```python
from build123d import *

# Parameters (mm, degrees)
SKETCH_1_W      = 56.1
SKETCH_1_H      = 8
SKETCH_1_R      = 1.5
EXTRUDE_1_DEPTH = 8
EXTRUDE_5_DEPTH = 8
EXTRUDE_6_DEPTH = 8


with BuildPart() as part:
    # 草图1 → 凸台-拉伸1 (new body)
    with BuildSketch(Plane.XY):
        with Locations((28.05, -4)):
            Rectangle(SKETCH_1_W, SKETCH_1_H)
        with Locations((5, -4)):
            Circle(SKETCH_1_R, mode=Mode.SUBTRACT)
        with Locations(Location((51.1, -4, 0), (0, 0, 180))):
            Circle(SKETCH_1_R, mode=Mode.SUBTRACT)
    extrude(amount=EXTRUDE_1_DEPTH)

    # 草图3 → 凸台-拉伸5 (add)
    with BuildSketch(Plane(origin=(0, 0, 0), x_dir=(-1, 0, 0), z_dir=(0, 0, -1))):
        with BuildLine():
            Line((-9.271136129, 3.747804008), (-22.014574203, 0))
            Line((-22.014574203, 0), (0, 0))
            ThreePointArc((0, 0), (250.320675472, 168.809291774), (500.641350944, 0))
            Line((500.641350944, 0), (509.912487072, 0))
            Line((509.912487072, 0), (509.912487072, 3.747804008))
            ThreePointArc((509.912487072, 3.747804008), (250.320675472, 178.809291774), (-9.271136129, 3.747804008))
        make_face()
    extrude(amount=-EXTRUDE_5_DEPTH)

    # 草图4 → 凸台-拉伸6 (add)
    with BuildSketch(Plane(origin=(0, 0, 0), x_dir=(-1, 0, 0), z_dir=(0, 0, -1))):
        with BuildLine():
            ThreePointArc((152.808242493, 161.280862452), (28.754408722, 106.028077563), (-56.1, 0))
            Line((-56.1, 0), (-39.057287102, 0))
            ThreePointArc((-39.057287102, 0), (9.399846723, 74.751796663), (83.727278113, 123.857375428))
            ThreePointArc((83.727278113, 123.857375428), (116.948632862, 145.004129758), (152.808242493, 161.280862452))
        make_face()
    extrude(amount=-EXTRUDE_6_DEPTH)


solid = part.part
```
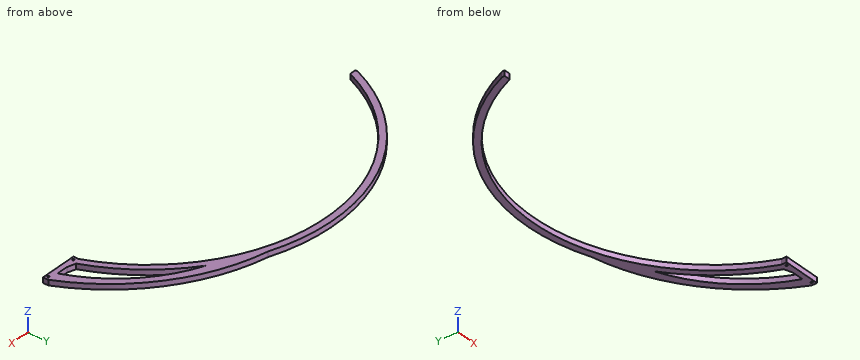
Read the model definition and answer for the solid it produces. Units are mm, in the model's axes. Give positions to 0.01 mm unless a question says otherwise; leave off trailing zeros. Order: outer loops, then holes, each group sorted by start corner. A loop starts at its lowest first (then second) coordinate and runs counter-clockwise, first axis right, second up.
(1) Find section D-D (y = 105). Give the vertices of the cut face in (x, z), plus the area to 3 significant figures.
(2) Find section B-B (y = 57). Give the vertices of the cut face in (x, z), plus the area to 3 significant figures.
(3) Find section A-A (z = 2.5). Give the vertices of the cut face in (x, y), plus the area to 3 significant figures.
(4) Given pin 1 (2.5 mm diameter, centred on y = -5.5, z = 4, fed in from -X); pin 2 (1 mm diameter, centred on y = 132.5, z = 4.5, fed in from +X); pin 3 (1.5 mm diameter, centred on y = 128.5, z = 6.5, fed in from -X); pin 4 (1.8 mm diameter, centred on x = 51.1, y = -4, fed in from +Z), each flat-ended and moving along its own axis, determine where each tip first touches the part or whether it passes through.
(5) Find section C-C (x = -88.5). Give the vertices of the cut face in (y, z), plus the area to 3 significant figures.
(6) Straight lines are drawn through the part: L1, parallel to X at y = 95.5, z = 3.75; L2, parallel to Y at x = 5, z = 4.75; L3, parallel to X at y = 50.5, z = 2. For each, find the intervals that lie inside material, in ascending order.
Result sheet:
1. outline: (-439.76, 0) - (-424.63, 0) - (-424.63, 8) - (-439.76, 8) - close; (-76.01, 0) - (-60.89, 0) - (-60.89, 8) - (-76.01, 8) - close; (-46.88, 0) - (-27.43, 0) - (-27.43, 8) - (-46.88, 8) - close
1. area: 398 mm2
2. outline: (-481.35, 0) - (-469.13, 0) - (-469.13, 8) - (-481.35, 8) - close; (-31.52, 0) - (-19.29, 0) - (-19.29, 8) - (-31.52, 8) - close; (6.38, 0) - (20.9, 0) - (20.9, 8) - (6.38, 8) - close
2. area: 312 mm2
3. outline: (-509.91, 0) - (-500.64, 0) arc R270 cw to (0, 0) - (0, -8) - (56.1, -8) - (56.1, 0) arc R287.5 ccw to (-152.81, 161.28) arc R280 ccw to (-509.91, 3.75) - close; hole (-83.73, 123.86) arc R280 cw to (9.27, 3.75) - (22.01, 0) - (39.06, 0) arc R217.85 ccw to start; hole circle Ø3 at (5, -4); hole circle Ø3 at (51.1, -4)
3. area: 9,840 mm2
4. pin 1: stops at x = 0
4. pin 2: stops at x = -68.9
4. pin 3: stops at x = -411.52
4. pin 4: passes through
5. outline: (114.94, 0) - (141.54, 0) - (141.54, 8) - (114.94, 8) - close
5. area: 213 mm2
6. L1: x = -449.6 to -435.29, -65.35 to -51.04, -33.19 to -15.9
6. L2: y = -8 to -5.5, -2.5 to 13.75, 58.71 to 75.41
6. L3: x = -485.67 to -473.68, -26.96 to -14.97, 11.35 to 25.9
